```python
from build123d import *

# Parameters (mm, degrees)
SM_BASE_FLANGE_1_DEPTH  = 80
HOLE_WIZARD_6_8_6_8_2_D = 6.8
CUT_EXTRUDE_3_DEPTH     = 5
MIRROR_5_COPY_1_D       = 6.8
MIRROR_5_COPY_2_DEPTH   = 5


# Sheet-metal steps are written as plain solids
with BuildPart() as part:
    # 草图3 → 基体-法兰1 (new body)
    with BuildSketch(Plane.XY):
        with BuildLine():
            Line((56, 0), (35.7366, 0))
            ThreePointArc((35.7366, 0), (35.215745145, 0.215745145), (35, 0.7366))
            Line((35, 0.7366), (35, 13.2634))
            ThreePointArc((35, 13.2634), (33.319788761, 17.319788761), (29.2634, 19))
            Line((29.2634, 19), (-29.2634, 19))
            ThreePointArc((-29.2634, 19), (-33.319788761, 17.319788761), (-35, 13.2634))
            Line((-35, 13.2634), (-35, 0.7366))
            ThreePointArc((-35, 0.7366), (-35.215745145, 0.215745145), (-35.7366, 0))
            Line((-35.7366, 0), (-56, 0))
            Line((-56, 0), (-56, -5))
            Line((-56, -5), (-35.7366, -5))
            ThreePointArc((-35.7366, -5), (-31.680211239, -3.319788761), (-30, 0.7366))
            Line((-30, 0.7366), (-30, 13.2634))
            ThreePointArc((-30, 13.2634), (-29.784254855, 13.784254855), (-29.2634, 14))
            Line((-29.2634, 14), (29.2634, 14))
            ThreePointArc((29.2634, 14), (29.784254855, 13.784254855), (30, 13.2634))
            Line((30, 13.2634), (30, 0.7366))
            ThreePointArc((30, 0.7366), (31.680211239, -3.319788761), (35.7366, -5))
            Line((35.7366, -5), (56, -5))
            Line((56, -5), (56, 0))
        make_face()
    extrude(amount=SM_BASE_FLANGE_1_DEPTH)

    # Ø6.8 (6.8) 直径孔2 (through all)
    with Locations(Plane(origin=(21, 19, 8.5), x_dir=(0, 0, 1), z_dir=(0, 1, 0))):
        with Locations((0, 0)):
            hole_wizard_6_8_6_8_2 = Hole(HOLE_WIZARD_6_8_6_8_2_D / 2)

    # 草图10 → 切除-拉伸3 (cut)
    with BuildSketch(Plane(origin=(0, 0, 0), x_dir=(1, 0, 0), z_dir=(0, 1, 0))):
        with BuildLine():
            Line((49.8, -52), (49.8, -72))
            ThreePointArc((49.8, -72), (46.3, -75.5), (42.8, -72))
            Line((42.8, -72), (42.8, -52))
            ThreePointArc((42.8, -52), (46.3, -48.5), (49.8, -52))
        make_face()
    cut_extrude_3 = extrude(amount=-CUT_EXTRUDE_3_DEPTH, mode=Mode.SUBTRACT)

    # 镜向4: Ø6.8 (6.8) 直径孔2, 切除-拉伸3 across plane
    add(hole_wizard_6_8_6_8_2.mirror(Plane(origin=(0, 0, 40), x_dir=(1, 0, 0), z_dir=(0, 0, -1))), mode=Mode.SUBTRACT)
    add(cut_extrude_3.mirror(Plane(origin=(0, 0, 40), x_dir=(1, 0, 0), z_dir=(0, 0, -1))), mode=Mode.SUBTRACT)

    # 镜向5: Ø6.8 (6.8) 直径孔2, 切除-拉伸3 across plane
    add(hole_wizard_6_8_6_8_2.mirror(Plane(origin=(0, 0, 0), x_dir=(0, 0, 1), z_dir=(1, 0, 0))), mode=Mode.SUBTRACT)
    add(cut_extrude_3.mirror(Plane(origin=(0, 0, 0), x_dir=(0, 0, 1), z_dir=(1, 0, 0))), mode=Mode.SUBTRACT)

    # 镜向5 copy 1 (through all)
    with Locations(Plane(origin=(-21, 19, 71.5), x_dir=(0, 0, -1), z_dir=(0, 1, 0))):
        with Locations((0, 0)):
            Hole(MIRROR_5_COPY_1_D / 2)

    # 镜向5 copy 2 sketch → 镜向5 copy 2 (cut)
    with BuildSketch(Plane(origin=(0, 0, 80), x_dir=(-1, 0, 0), z_dir=(0, 1, 0))):
        with BuildLine():
            Line((49.8, -52), (49.8, -72))
            ThreePointArc((49.8, -72), (46.3, -75.5), (42.8, -72))
            Line((42.8, -72), (42.8, -52))
            ThreePointArc((42.8, -52), (46.3, -48.5), (49.8, -52))
        make_face()
    extrude(amount=-MIRROR_5_COPY_2_DEPTH, mode=Mode.SUBTRACT)


solid = part.part
```
Part model, mm, in its own coordinate system. A direction names the side the tool comes from. Round coordinates to 2 decimals unless told otherwise and drop trailing zeros. Write each loop counter-clockwise with the first axis right and the second up, starting at its lowest first coordinate (ties: lowest second). Pieces come first, ordered by that corner, then holes. Notation, with made-up numbers: M 48.25,-23 L 74.25,-23 A31 ccw 74.25,6 Z; hole C 82.5,84 d5. An arc over 180 degrees is marked long. Answer as CSV lines item,"result". Start each with the question number.
1) Band-saw the part on A-A (z = 58). List the corners of the cut face in (x, y), then the cut area to 3 significant figures.
2) Band-saw the part on C-C (y = -2.5). List the corners of the cut face in (x, z), then the cut area to 3 significant figures.
3) Which spindle directions (+Z, -Z, +X, -X, +Y, -Y) get a long thin tool onto all of the face, cutting with end or side? Do faces 1 (the face through (35, 7, 39)), 2 (the face through (-46.4, -2.5, 75.5)), 3 (the face through (0, 14, 39)). Say none if no direction does.
4) Drop flat-ended pins along their axis: pin 1 (1.5 mm diameter, centred on y = 13.5, z = 24.5, fed in from -X); pin 2 (10 mm diameter, centred on x = -50, z = 44.5, fed in from +Y); pin 3 (4 mm diameter, centred on x = -21, z = 8.5, fed in from +Y); pin 4 (11 mm diameter, centred on x = 21, z = 71.5, fed in from -Y). Give the stop position or say it passes through.
5) Band-saw the part on B-B (y = 10.75). List the corners of the cut face in (x, z).
6) Band-saw the part on D-D (x = 46.3). List the corners of the cut face in (y, z).
7) Drill centre lines: L1, parallel to X at y = 16.05, z = 8.5; L2, parallel to X at y = 4.75, z = 36; L3, parallel to Y at x = 36.5, z = 54.5. Where is each one in solid material? Low to high.
Worked out:
1,outline,"M -56,-5 L -49.8,-5 L -49.8,0 L -56,0 Z; M -42.8,-5 L -35.74,-5 A5.74 ccw -30,0.74 L -30,13.26 A0.74 cw -29.26,14 L 29.26,14 A0.74 cw 30,13.26 L 30,0.74 A5.74 ccw 35.74,-5 L 42.8,-5 L 42.8,0 L 35.74,0 A0.74 cw 35,0.74 L 35,13.26 A5.74 ccw 29.26,19 L -29.26,19 A5.74 ccw -35,13.26 L -35,0.74 A0.74 cw -35.74,0 L -42.8,0 Z; M 49.8,-5 L 56,-5 L 56,0 L 49.8,0 Z"
1,area,"652 mm²"
2,outline,"M -56,0 L -31,0 L -31,80 L -56,80 Z; M 31,0 L 56,0 L 56,80 L 31,80 Z; hole M -49.8,8 A3.5 ccw -42.8,8 L -42.8,28 A3.5 ccw -49.8,28 Z; hole M -49.8,52 A3.5 ccw -42.8,52 L -42.8,72 A3.5 ccw -49.8,72 Z; hole M 42.8,8 A3.5 ccw 49.8,8 L 49.8,28 A3.5 ccw 42.8,28 Z; hole M 42.8,52 A3.5 ccw 49.8,52 L 49.8,72 A3.5 ccw 42.8,72 Z"
2,area,"3,290 mm²"
3,face 1,"+Z, -Z, +X, +Y"
3,face 2,"+Y, -Y"
3,face 3,"+Z, -Z, -Y"
4,pin 1,"x = -35"
4,pin 2,"y = 0"
4,pin 3,"through"
4,pin 4,"y = 14"
5,outline,"M -35,0 L -30,0 L -30,80 L -35,80 Z; M 30,0 L 35,0 L 35,80 L 30,80 Z"
6,outline,"M -5,0 L 0,0 L 0,4.5 L -5,4.5 Z; M -5,31.5 L 0,31.5 L 0,48.5 L -5,48.5 Z; M -5,75.5 L 0,75.5 L 0,80 L -5,80 Z"
7,L1,"-34.28 to -24.4, -17.6 to 17.6, 24.4 to 34.28"
7,L2,"-35 to -30, 30 to 35"
7,L3,"-5 to 0"
